Read the model definition and answer for the solid it produces. Units are mm, in the model's axes. Give positions to 0.01 mm unless a question says otherwise; leave off trailing zeros. Put each result on its own line as item: value. Start each with the question number.
1. For a pull along Y with two mould halves and no side action, classify faces 1 (the cylindrical face through (3.3, 13.1, -0.2)), 2 (the cylindrical face through (13.73, 43.61, -0.18)), 3 (the cylindrical face through (-9.702, 9.407, -0.218)) as released by +Y, released by -Y, zero draft, split by the parting line, or undercut.
2. A cutting plane is placed at A-A, the plane z = -11. Count the separate pieces of the cut face and the enclosed holes in it, plus the area to 3 significant figures.
3. Consider L1, parallel to X at y = -11, z = 12; L2, parallel to X at y = 37.5, z = 9; L3, parallel to X at y = -26.5, z = -6. Determine where each line is inside the solid, lowest interval first. Write a range as from..to.
4. Given pin 1 Ø9.5 at (y, z) = (-23.5, 1) entering from +X; pin 2 Ø5 at (x, y) = (34.5, -32) entering from -Z; pin 3 Ø1 at (x, z) = (21.5, -10.5) entering from +Y; pin 4 Ø1.5 at (x, z) = (-2, -6) entering from -Y, each flat-ended and moving along its own axis, determine where each tip first touches the part or whether it passes through.
Autodesk Inventor part; units mm, degrees
ref_plane "YZ Plane" through (0, 0, 0) normal (1, 0, 0) x (0, 1, 0)
ref_plane "XZ Plane" through (0, 0, 0) normal (0, 1, 0) x (-1, 0, 0)
ref_plane "XY Plane" through (0, 0, 0) normal (0, 0, 1) x (1, 0, 0)
sketch "Sketch1" plane through (0, 0, 0) normal (1, 0, 0) x (0, 1, 0)
  line L0 (0, 15.5575) -> (45.72, 15.5575)
  line L1 (45.72, 15.5575) -> (45.72, -15.5575)
  line L2 (45.72, -15.5575) -> (0, -15.5575)
  line L3 (0, -15.5575) -> (0, 15.5575)
  arc A0 (45.72, 13.0175) -> (45.72, 15.5575) centre (45.72, 14.2875) ccw
  arc A1 (45.72, -15.5575) -> (45.72, -13.0175) centre (45.72, -14.2875) ccw
  line L4 (45.72, 13.0175) -> (50.8, 13.0175)
  line L5 (50.8, 13.0175) -> (50.8, -13.0175)
  line L6 (50.8, -13.0175) -> (45.72, -13.0175)
  line L7 (45.72, -13.0175) -> (45.72, 13.0175)
  point P0 (0, 0)
  point P1 (45.72, 0)
  point P2 (0, 0)
  dimension "d0" = 1.27
  dimension "d1" = 1.27
  dimension "d2" = 45.72
  dimension "d3" = 26.035
  dimension "d4" = 5.08
revolve "Revolution1" add sketch "Sketch1" angle 360 about axis through (0, 0, -15.5575) along (0, 0, 1) contours L0 L1 L2 L3 | A0 L1 | L1 A1
sketch "Sketch2" plane through (0, 0, 15.5575) normal (0, 0, 1) x (1, 0, 0)
  line L0 (-6.35, 3.6662) -> (0, 7.3323)
  line L1 (0, 7.3323) -> (6.35, 3.6662)
  line L2 (6.35, 3.6662) -> (6.35, -3.6662)
  line L3 (6.35, -3.6662) -> (0, -7.3323)
  line L4 (0, -7.3323) -> (-6.35, -3.6662)
  line L5 (-6.35, -3.6662) -> (-6.35, 3.6662)
  point P0 (0, 0)
  point P1 (0, 0)
  point P2 (6.35, 0)
  dimension "d6" = 12.7
extrude "Extrusion1" cut sketch "Sketch2" against normal through all
sketch "Sketch3" plane through (0, 0, 15.5575) normal (0, 0, 1) x (1, 0, 0)
  circle A0 centre (0, 0) radius 12.5
  circle A1 centre (0, 0) radius 45.72 construction
  circle A2 centre (0, 0) radius 40.72
  line L0 (0, -12.5) -> (0, -40.72)
  line L1 (6.35, -3.6662) -> (0, -7.3323)
  line L2 (0, -7.3323) -> (-6.35, -3.6662)
  line L3 (-6.35, -3.6662) -> (-6.35, 3.6662)
  line L4 (-6.35, 3.6662) -> (0, 7.3323)
  line L5 (0, 7.3323) -> (6.35, 3.6662)
  line L6 (6.35, 3.6662) -> (6.35, -3.6662)
  circle A3 centre (0, 0) radius 45.72
  line L7 (0, 0) -> (35.2646, -20.36)
  line L8 (0, 0) -> (35.2646, 20.36)
  line L9 (0, 0) -> (0, 40.72)
  line L10 (0, 0) -> (-35.2646, 20.36)
  line L11 (0, 0) -> (-35.2646, -20.36)
  line L12 (-11.8566, 3.9587) -> (-36.448, 18.1565)
  line L13 (-9.3566, 8.2888) -> (-33.948, 22.4867)
  line L14 (-11.8566, -3.9587) -> (-36.448, -18.1565)
  line L15 (-9.3566, -8.2888) -> (-33.948, -22.4867)
  line L16 (-2.5, -12.2474) -> (-2.5, -40.6432)
  line L17 (2.5, -12.2474) -> (2.5, -40.6432)
  line L18 (9.3566, -8.2888) -> (33.948, -22.4867)
  line L19 (11.8566, -3.9587) -> (36.448, -18.1565)
  line L20 (11.8566, 3.9587) -> (36.448, 18.1565)
  line L21 (9.3566, 8.2888) -> (33.948, 22.4867)
  line L22 (2.5, 12.2474) -> (2.5, 40.6432)
  line L23 (-2.5, 12.2474) -> (-2.5, 40.6432)
  point P0 (-36.448, -18.1565)
  dimension "d9" = 25
  dimension "d10" = 5
  dimension "d13" = 2.5
  dimension "d14" = 5
  dimension "d17" = 360
extrude "Extrusion2" cut sketch "Sketch3" against normal through all contours A0 L20 A2 L19 | A0 L22 A2 L21 | L18 A2 L17 A0 | A0 L13 A2 L23 | L16 A2 L15 A0 | A0 L14 A2 L12
fillet "Fillet1" radius 5 2 edges at (-33.948, 22.4867, 0) (-36.448, 18.1565, 0)
pattern_circular "Circular Pattern1" count 6 over 360 about axis through (0, 0, -10) along (0, 0, 1) of "Fillet1"
fillet "Fillet2" radius 5 2 edges at (9.3566, 8.2888, 0) (11.8566, 3.9587, 0)
pattern_circular "Circular Pattern2" count 6 over 360 about axis through (0, 0, -10) along (0, 0, 1) of "Fillet2"
equation "\"d1\" = d0"
properties part number "CUSTOM 4IN WHEEL" material "Aluminum 6061"
Return value:
1. face 1: undercut
1. face 2: split by the parting line
1. face 3: undercut
2. separate pieces: 1
2. enclosed holes: 7
2. area: 2,680 mm2
3. L1: x = -44.38..-39.21, -24.05..-14.05, -5.94..5.94, 14.05..24.05, 39.21..44.38
3. L2: x = -26.15..-15.87, -3.21..3.21, 15.87..26.15
3. L3: x = -37.26..-30.8, -2.5..2.5, 30.8..37.26
4. pin 1: stops at x = 41.7
4. pin 2: stops at z = -15.56
4. pin 3: stops at y = 40.61
4. pin 4: stops at y = -45.7
